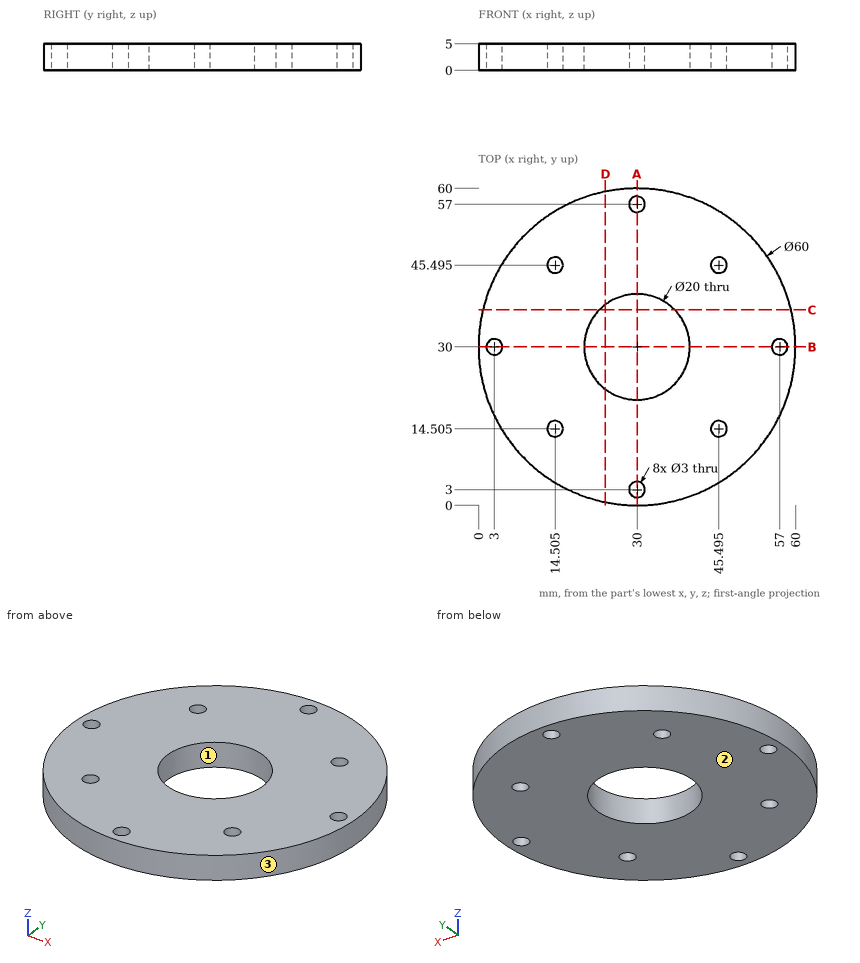
Geometry check sheet. Reference: drawing and pictorial views, mm from the part's lowest x, y, z. Coordinates: 2 decimals unless noted, no trailing zeros. Loops run counter-clockwise (first coordinate to the right, second up) from the corner with the lowest first, then second, coordinate; pieces in that order, holes last. Notation, with made-up numbers: M -27,3.5 L 10,3.5 A20 ccw 10,13.5 Z; hole C -23.5,33 d5. An arc over 180 degrees is marked long. One line per item, written item: value.
1. Mould release check, pull along X, two halves, no side actions. Record for the marked faces 1, 2 and 3: pulls with the +X half, pulls with the -X half, needs draft (parallel to the pull), parting line crosses it, or undercut.
Answers follow:
face 1: undercut
face 2: needs draft
face 3: parting line crosses it
2. Material ranges on line 1 along Y through (x, z) = (30, 3.85); line 2 along Y through (x, z) = (29.5, 2.25); line 3 along X through (y, z) = (46, 3.9), recorded low to high. Write a range as from..to.
Answers follow:
line 1: 0..1.5, 4.5..20, 40..55.5, 58.5..60
line 2: 0..1.59, 4.41..20.01, 39.99..55.59, 58.41..60
line 3: 4.62..13.09, 15.92..44.08, 46.91..55.38
3. Gauge pin test, flat ends, axial feed: P1, Ø1.5, axis at y = 45.5, z = 2.5, coming from the +X side; P2, Ø2.5, axis at x = 45.495, y = 14.505, coming from the -Z side; P3, Ø1, axis at x = 48, z = 1.5, coming from the -Y side; P4, Ø1, axis at x = 40, z = 3, coming from the +Y side. Record the tip position at first contact, or that the pin passes through.
Answers follow:
P1: x = 56.12
P2: through
P3: y = 5.63
P4: y = 58.46
4. Section check D-D on x = 24. Record the cut outline in (y, z).
Answers follow:
outline: M 0.61,0 L 22,0 L 22,5 L 0.61,5 Z; M 38,0 L 59.39,0 L 59.39,5 L 38,5 Z
5. Section check C-C on y = 37. Record the cut outline in (x, z), plus the area to 3 significant figures.
Answers follow:
outline: M 0.83,0 L 22.86,0 L 22.86,5 L 0.83,5 Z; M 37.14,0 L 59.17,0 L 59.17,5 L 37.14,5 Z
area: 220 mm^2
6. Section check A-A on x = 30. Record the cut outline in (y, z), plus the area to 3 significant figures.
Answers follow:
outline: M 0,0 L 1.5,0 L 1.5,5 L 0,5 Z; M 4.5,0 L 20,0 L 20,5 L 4.5,5 Z; M 40,0 L 55.5,0 L 55.5,5 L 40,5 Z; M 58.5,0 L 60,0 L 60,5 L 58.5,5 Z
area: 170 mm^2
